Design review of the part built by this model. Coordinates are the model's own, in mm. Face numbers are marked on the shaded views. A direction names the side the tool comes from. Round coordinates to 2 decimals unless told otherwise and drop trailing zeros. Loops run counter-clockwise (first coordinate to the right, second up) from the corner with the lowest first, then second, coordinate; pieces in that order, holes last. Notation, with made-up numbers: (1, 63) - (6, 63) arc R17 ccw to (6, 80) - close; hole circle Ø1 at (-3.75, 11.5). An arc over 180 degrees is marked (long way). Answer as CSV lines item,"result". Start each with the question number.
(1) Mouldability with a two-part tool opening along Y and no side actions: class the marked faces 3, 4, 5 and 6 as released by +Y, released by -Y, zero draft, split by the parting line, or undercut.
(2) For P1, Ø0.6, axis at x = 0.5, z = -2, coming from the +Y side; P2, Ø5, axis at x = -4, z = 0.5, coming from the +Y side; P3, Ø4, axis at y = -1.5, z = 17, coming from the -X side, all flat-tipped, find the tip position at first contact; note any pin that passes through.
(3) For the marked faces 1 and 2, list the 3-axis set-ups (+Z, -Z, +X, -X, +Y, -Y) from which the entire face can be reached by the end or side of a thin tool; tool diameter is ignored.
(4) Wall thickness on L1, parallel to Z at x = 0.75, y = 4.5; L2, parallel to Z at x = -0.25, y = -4; L3, parallel to Y at x = 0, z = 7.5: over which ranges is each line inside the solid? List them lowest first.
(5) Consider section A-A (x = 0). Give the boundary of the cut face in (y, z), and give its area (3 significant figures).
(6) Consider section D-D (x = 3.25). Give the boundary of the cut face in (y, z).
(7) Consider section B-B (y = -2.5). Give the boundary of the cut face in (x, z).
(8) Consider section C-C (z = 2). Give the boundary of the cut face in (x, y), and give its area (3 significant figures).
from build123d import *

# Parameters (mm, degrees)
S01_M6_SHANK_R                   = 3
F_01_M6_SHANK_DEPTH              = 20
F_02_START                       = -1.2
S02_HEAD_SEATING_DIAMETER_R      = 5.25
F_02_HEAD_SEATING_DIAMETER_DEPTH = 1.2
F_03_START                       = -3.3
S03_BUTTON_CROWN_R               = 4.3
F_03_BUTTON_CROWN_DEPTH          = 2.1
F_04_START                       = -3.4
F_04_4_MM_HEX_KEY_DEPTH          = 2.2


with BuildPart() as part:
    # S01 - M6 shank → 01 - M6 shank (new body)
    with BuildSketch(Plane.XY):
        Circle(S01_M6_SHANK_R)
    extrude(amount=F_01_M6_SHANK_DEPTH)

    # S02 - Head seating diameter → 02 - Head seating diameter (add)
    with BuildSketch(Plane.XY.offset(F_02_START)):
        Circle(S02_HEAD_SEATING_DIAMETER_R)
    extrude(amount=F_02_HEAD_SEATING_DIAMETER_DEPTH)

    # S03 - Button crown → 03 - Button crown (add)
    with BuildSketch(Plane.XY.offset(F_03_START)):
        Circle(S03_BUTTON_CROWN_R)
    extrude(amount=F_03_BUTTON_CROWN_DEPTH)

    # S04 - 4 mm hex key → 04 - 4 mm hex key (cut)
    with BuildSketch(Plane.XY.offset(F_04_START)):
        Polygon((2.309401077, 0), (1.154700538, 2), (-1.154700538, 2), (-2.309401077, 0), (-1.154700538, -2), (1.154700538, -2), align=None)
    extrude(amount=F_04_4_MM_HEX_KEY_DEPTH, mode=Mode.SUBTRACT)


solid = part.part
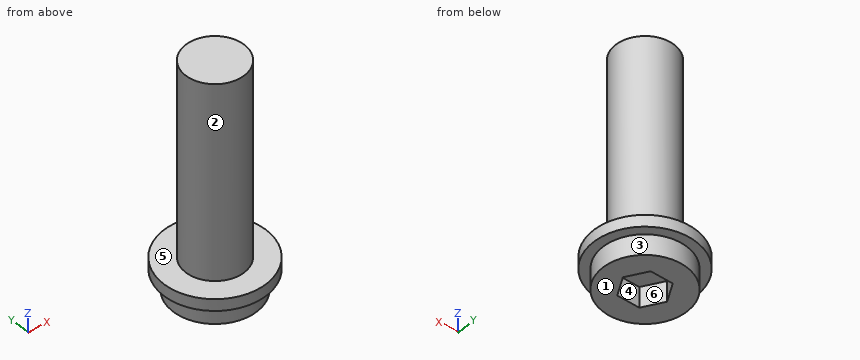
Determined:
1,face 3,"split by the parting line"
1,face 4,"undercut"
1,face 5,"zero draft"
1,face 6,"undercut"
2,P1,"stops at y = 4.3"
2,P2,"stops at y = 5.02"
2,P3,"stops at x = -3"
3,face 1,"-Z, +X, -X, +Y, -Y"
3,face 2,"+Z"
4,L1,"z = -1.2 to 0"
4,L2,"z = -3.3 to 0"
4,L3,"y = -3 to 3"
5,outline,"(-5.25, -1.2) - (-4.3, -1.2) - (-4.3, -3.3) - (-2, -3.3) - (-2, -1.2) - (2, -1.2) - (2, -3.3) - (4.3, -3.3) - (4.3, -1.2) - (5.25, -1.2) - (5.25, 0) - (3, 0) - (3, 20) - (-3, 20) - (-3, 0) - (-5.25, 0) - close"
5,area,"142 mm^2"
6,outline,"(-4.12, -1.2) - (-2.82, -1.2) - (-2.82, -3.3) - (2.82, -3.3) - (2.82, -1.2) - (4.12, -1.2) - (4.12, 0) - (-4.12, 0) - close"
7,outline,"(-4.62, -1.2) - (-3.5, -1.2) - (-3.5, -3.3) - (3.5, -3.3) - (3.5, -1.2) - (4.62, -1.2) - (4.62, 0) - (1.66, 0) - (1.66, 20) - (-1.66, 20) - (-1.66, 0) - (-4.62, 0) - close"
8,outline,"circle Ø6 at (0, 0)"
8,area,"28.3 mm^2"
